Can you work these out from the model? Positions are in its coordinate system, mm. A direction names the side the tool comes from. Coordinates: 2 decimals unless noted, no trailing zeros. Loops run counter-clockwise (first coordinate to the right, second up) from the corner with the lowest first, then second, coordinate; pieces in that order, holes last. Notation, with made-up numbers: (-33, 55) - (1, 55) arc R24 cw to (1, 88) - close; hole circle Ø10 at (-25, 15). An arc over 180 degrees is marked (long way). Put each result on its own line as item: value. Start each with the question number.
Autodesk Inventor part; units mm, degrees
ref_plane "YZ Plane" through (0, 0, 0) normal (1, 0, 0) x (0, 1, 0)
ref_plane "XZ Plane" through (0, 0, 0) normal (0, 1, 0) x (-1, 0, 0)
ref_plane "XY Plane" through (0, 0, 0) normal (0, 0, 1) x (1, 0, 0)
sketch "Szkic1" plane through (0, 0, 0) normal (0, 1, 0) x (-1, 0, 0)
  circle A0 centre (0, 0) radius 13.5
  dimension "d0" = 27
extrude "Wyciągnięcie proste1" add sketch "Szkic1" along normal blind 1
sketch "Szkic2" plane through (0, 1, 0) normal (0, 1, 0) x (1, 0, 0)
  circle A0 centre (0, 0) radius 12.5
  dimension "d3" = 25
extrude "Wyciągnięcie proste2" add sketch "Szkic2" along normal blind 4
sketch "Szkic3" plane through (0, 5, 0) normal (0, 1, 0) x (1, 0, 0)
  arc A0 (2.12, 1.59) -> (2.12, -1.59) centre (0, 0) ccw
  line L0 (2.12, -1.59) -> (2.12, 1.59)
  dimension "d6" = 5.3
  dimension "d7" = 2.12
extrude "Wyciągnięcie proste3" cut sketch "Szkic3" against normal through all
sketch "Szkic4" plane through (0, 5, 0) normal (0, 1, 0) x (1, 0, 0)
  circle A0 centre (0, -6.75) radius 3
  point P0 (0, 0)
  dimension "d10" = 6
extrude "Wyciągnięcie proste4" cut sketch "Szkic4" against normal blind 2.5
sketch "Szkic5" plane through (0, 2.5, 6.75) normal (0, 1, 0) x (1, 0, 0)
  circle A0 centre (0, 0) radius 1.6
  point P0 (0, 6.75)
  dimension "d13" = 3.2
extrude "Wyciągnięcie proste5" cut sketch "Szkic5" against normal blind 3.5
pattern_circular "Szyk kołowy1" count 2 over 360 about axis through (0, 1, 0) along (0, 1, 0) of "Wyciągnięcie proste4", "Wyciągnięcie proste5"
sketch "Szkic6" plane through (0, 5, 0) normal (0, 1, 0) x (1, 0, 0)
  circle A0 centre (0, 0) radius 11
  circle A1 centre (0, 6.75) radius 3
  circle A2 centre (0, 6.75) radius 3
  circle A3 centre (0, -6.75) radius 3
  circle A4 centre (0, -6.75) radius 3
  arc A5 (2.12, 1.59) -> (2.12, -1.59) centre (0, 0) ccw
  line L0 (2.12, 1.59) -> (2.12, -1.59)
  line L1 (2.12, -1.59) -> (2.12, 1.59)
  dimension "d19" = 22
extrude "Wyciągnięcie proste6" add sketch "Szkic6" along normal blind 3
sketch "Szkic7" plane through (0, 8, 0) normal (0, 1, 0) x (1, 0, 0)
  arc A0 (2.12, 1.59) -> (2.12, -1.59) centre (0, 0) ccw
  line L0 (2.12, 1.59) -> (2.12, -1.59)
  line L1 (2.12, -1.59) -> (2.12, 1.59)
extrude "Wyciągnięcie proste7" add sketch "Szkic7" against normal blind 0.5
properties part number "_Drukowanie 3D"
Q1. I want a section at B-B on z = 6.75. List the corners of the cut face in (x, y) for me.
Q2. We'd pull the mould along X, two halves only. Please class faces 4 (the flat face through (1.3, 2.5, 8)), 5 (the cylindrical face through (11.923, 2.972, 3.755)), 6 (the flat face through (0, 8, 0)), 7 (the cylindrical face through (-2.65, 3.7, 0.09)): released by +X, released by -X, zero draft, split by the parting line, or undercut.
Q3. I want a section at D-D on x = 5.25. List the corners of the cut face in (y, z) for me.
Q4. I want a section at C-C on y = 4.5. List the corners of the cut face in (x, z) for me.
Q5. Will these pins go through, and if not, where does the flat tip stop? pin 1 (3.5 mm diameter, centred on x = 0, z = 6.75, fed in from +Y); pin 2 (1 mm diameter, centred on x = -9.5, y = 6.5, fed in from -Z); pin 3 (2 mm diameter, centred on y = 2.5, z = 2.5, fed in from +X).
Q6. I want a section at A-A on x = 0. Count the separate pieces of the cut face and the enclosed holes in it, and give its area (4 significant figures).
Q7. Please list where these lines run through material, in increasing order: line 1 along Z through (x, y) = (0, 4.5); line 2 along Z through (x, y) = (0, 0.8); line 3 along X through (y, z) = (4, 0). Write a range as [from, to].
Q8. On a 3-axis mill with a long thin cutter (end or side, diameter ignored), from which of +Z, -Z, +X, -X, +Y, -Y can I reach the whole of each face in a straight line? I mean faces 1 (the flat face through (2.12, 4, 0)), 2 (the flat face through (5, 5, 10)), 3 (the flat face through (-3, 0, 0)). Say none if no direction works.
Calculated:
1. outline: (-11.69, 0) - (-1.6, 0) - (-1.6, 2.5) - (-3, 2.5) - (-3, 8) - (-8.69, 8) - (-8.69, 5) - (-10.52, 5) - (-10.52, 1) - (-11.69, 1) - close; (1.6, 0) - (11.69, 0) - (11.69, 1) - (10.52, 1) - (10.52, 5) - (8.69, 5) - (8.69, 8) - (3, 8) - (3, 2.5) - (1.6, 2.5) - close
2. face 4: undercut
2. face 5: split by the parting line
2. face 6: zero draft
2. face 7: undercut
3. outline: (0, -12.44) - (1, -12.44) - (1, -11.34) - (5, -11.34) - (5, -9.67) - (8, -9.67) - (8, 9.67) - (5, 9.67) - (5, 11.34) - (1, 11.34) - (1, 12.44) - (0, 12.44) - close
4. outline: circle Ø25 at (0, 0); hole circle Ø6 at (0, -6.75); hole circle Ø6 at (0, 6.75); hole (2.12, -1.59) - (2.12, 1.59) arc R2.65 ccw (long way) to start
5. pin 1: y = 2.5
5. pin 2: z = -6.32
5. pin 3: x = 12.41
6. separate pieces: 3
6. enclosed holes: 0
6. area: 71.25 mm2
7. line 1: [-12.5, -9.75], [-3.75, -2.65], [2.65, 3.75], [9.75, 12.5]
7. line 2: [-13.5, -8.35], [-5.15, -2.65], [2.65, 5.15], [8.35, 13.5]
7. line 3: [-12.5, -2.65], [2.12, 12.5]
8. face 1: -Y
8. face 2: +Y
8. face 3: +Z, -Z, +X, -X, -Y
